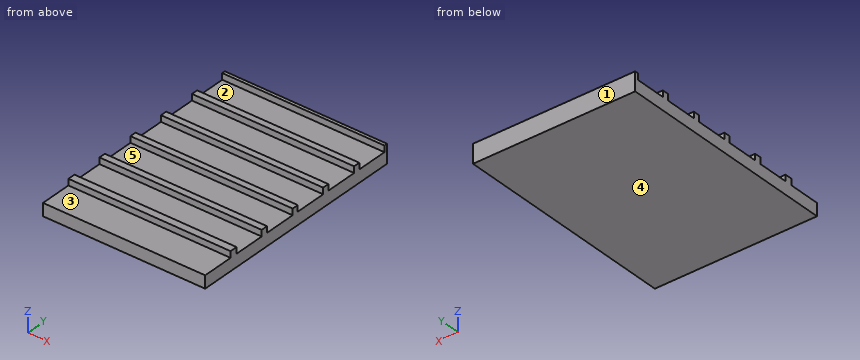
```python
from build123d import *

# Parameters (mm, degrees)
F0_W      = 129.826464
F0_H      = 180.507004
F1_DEPTH  = 15
F2_W      = 129.826464
F2_H      = 25.231384
F4_DEPTH  = 5
F3_W      = 129.826464
F3_H      = 24.901012
F5_DEPTH  = 5
F7_W      = 193.91631
F7_H      = 25.443339
F8_DEPTH  = 5
F9_W      = 129.826464
F9_H      = 24.94248
F9_H_2    = 25.64016
F9_H_3    = 25.21283
F10_DEPTH = 5


with BuildPart() as f1:
    # F0 (on Top) → F1 (new body)
    with BuildSketch(Plane.XY):
        with Locations((-4.98702, 25.216296)):
            Rectangle(F0_W, F0_H)
    extrude(amount=F1_DEPTH)

    # F2 (on face) → F4 (cut)
    with BuildSketch(Plane.XY.offset(15)):
        with Locations((-4.98702, -52.421514)):
            Rectangle(F2_W, F2_H)
    extrude(amount=-F4_DEPTH, mode=Mode.SUBTRACT)

    # F3 (on face) → F5 (cut)
    with BuildSketch(Plane.XY.offset(15)):
        with Locations((-4.98702, -21.404932)):
            Rectangle(F3_W, F3_H)
    extrude(amount=-F5_DEPTH, mode=Mode.SUBTRACT)

    # F7 (on face) → F8 (cut)
    with BuildSketch(Plane.XY.offset(15)):
        with Locations((10.563256, 9.04997)):
            Rectangle(F7_W, F7_H)
    extrude(amount=-F8_DEPTH, mode=Mode.SUBTRACT)

    # F9 (on face) → F10 (cut)
    with BuildSketch(Plane.XY.offset(15)):
        with Locations((-4.98702, 100.438904)):
            Rectangle(F9_W, F9_H)
        with Locations((-4.98702, 70.019551)):
            Rectangle(F9_W, F9_H_2)
        with Locations((-4.98702, 39.465022)):
            Rectangle(F9_W, F9_H_3)
    extrude(amount=-F10_DEPTH, mode=Mode.SUBTRACT)


solid = f1.part
```
CAD build for the part. Positions are in the model's coordinates, mm. Face numbers are marked on the shaded views. A direction names the side the tool comes from. Coordinates: 2 decimals unless noted, no trailing zeros. Order: outer loops, then holes, each group sorted by start corner. A loop starts at its lowest first (then second) coordinate and runs counter-clockwise, first axis right, second up. Notation, with made-up numbers: M -22.75,25 L 14.25,25 A20 ccw 14.25,61 Z; hole C 75,-14.5 d3. An arc over 180 degrees is marked long. Write each question's results on one line, items separated by ' | '. Start each with the question number.
Q1. Which spindle directions (+Z, -Z, +X, -X, +Y, -Y) get a long thin tool onto all of the face, cutting with end or side? Do the marked faces 4 and 5. Say none if no direction does.
Q2. Cut at A-A (x = 12.5). List the corners of the cut face in (y, z), then the cut area to 3 significant figures.
Q3. Drill centre lines: probe 1 along Y at (x, z) = (-24, 14); probe 2 along Z at (x, y) = (-30, -55). Where is each one in solid material? Low to high. Write a range as from..to.
Q4. Flat gauge pins, fed straight in: P1, Ø5.5, axis at x = 15, z = 13, coming from the -Y side; P2, Ø7.5, axis at x = -4, y = 104.5, coming from the +Z side. Where does each tip first touch, or does it go through?
Q5. Pull direction Y, two halves, no side cores. Call the marked faces 1, 2 and 3: +Y half, -Y half, draft (parallel to the pull), parting line (faces both ways), or undercut.
Q6. Cut at B-B (y = 4). List the corners of the cut face in (x, z), then the cut area to 3 significant figures.
Found:
1) face 4: -Z, +X, -X, +Y, -Y | face 5: +Z, +X, -X
2) outline: M -65.04,0 L 115.47,0 L 115.47,15 L 112.91,15 L 112.91,10 L 87.97,10 L 87.97,15 L 82.84,15 L 82.84,10 L 57.2,10 L 57.2,15 L 52.07,15 L 52.07,10 L 26.86,10 L 26.86,15 L 21.77,15 L 21.77,10 L -3.67,10 L -3.67,15 L -8.95,15 L -8.95,10 L -33.86,10 L -33.86,15 L -39.81,15 L -39.81,10 L -65.04,10 Z | area: 1,950 mm²
3) probe 1: -39.81..-33.86, -8.95..-3.67, 21.77..26.86, 52.07..57.2, 82.84..87.97, 112.91..115.47 | probe 2: 0..10
4) P1: y = -39.81 | P2: z = 10
5) face 1: +Y half | face 2: undercut | face 3: draft
6) outline: M -69.9,0 L 59.93,0 L 59.93,10 L -69.9,10 Z | area: 1,300 mm²
